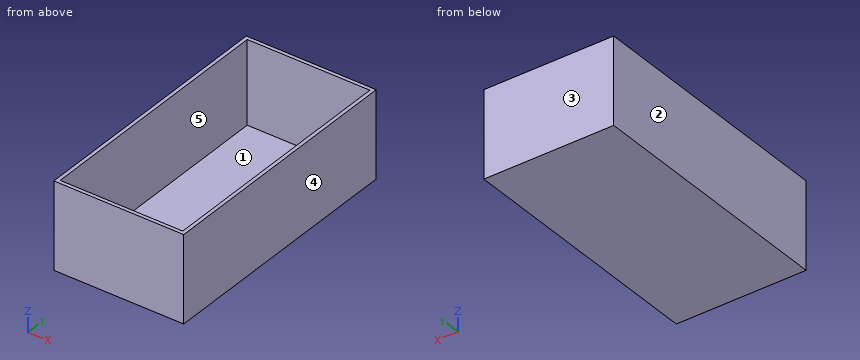
Autodesk Inventor part; units mm, degrees
ref_plane "YZ Plane" through (0, 0, 0) normal (1, 0, 0) x (0, 1, 0)
ref_plane "XZ Plane" through (0, 0, 0) normal (0, 1, 0) x (-1, 0, 0)
ref_plane "XY Plane" through (0, 0, 0) normal (0, 0, 1) x (1, 0, 0)
sketch "grey cabinet" plane through (0, 0, 0) normal (0, 1, 0) x (-1, 0, 0)
  line L0 (914.4, 609.6) -> (0, 609.6)
  line L1 (0, 609.6) -> (0, 0)
  line L2 (0, 0) -> (914.4, 0)
  line L3 (914.4, 0) -> (914.4, 609.6)
  dimension "d0" = 914.4
  dimension "d1" = 609.6
extrude "grey cabinet2" add sketch "grey cabinet" along normal blind 1828.8
shell "Shell1" thickness 25.4 removed faces 1 at (-609.6, 609.6, 609.6)
properties part number "grey cabinet"
Can you work these out from the model? Positions are in its coordinate system, mm. Face numbers are marked on the shaded views. A direction names the side the tool comes from. Round coordinates to 2 decimals unless told otherwise and drop trailing zeros. Loops run counter-clockwise (first coordinate to the right, second up) from the corner with the lowest first, then second, coordinate; pieces in that order, holes last. Notation, with made-up numbers: (-7, 49.25) -> (46, 49.25) arc R20 ccw to (46, 60.25) -> close; hole circle Ø7 at (-39, 52). An arc over 180 degrees is marked (long way). One line per item, written item: value. Start each with the question number.
1. If we section it at C-C, the plane x = -718: Write out the boundary of the cut face in (y, z), then the cut area to 3 significant figures.
2. If we section it at A-A, the plane z = 543.5: Write out the boundary of the cut face in (x, y).
3. If I drill on probe 1 along X at (y, z) = (388.5, 225.5); probe 2 along Y at (x, z) = (-160.5, 513); probe 3 along Z at (x, y) = (-839.5, 1678), over which ranges is the centre line in solid material (lowest first)?
4. If we section it at B-B, the plane y = 1454: Write out the boundary of the cut face in (x, z), then the cut area to 3 significant figures.
5. If we mould it in two halves opening along Y, with no side actions, what happens to the marked faces 1, 2 and 3? For each: pulls with the +Y half, pulls with the -Y half, needs draft (parallel to the pull), parting line crosses it, or undercut.
6. For pin 1 (5 mm diameter, centred on x = -574, z = 324, fed in from -Y), with a flat end and sliding along its axis, tell me the tip position at first contact or that it passes through.
7. For the marked faces 4 and 5, which set-ups out of +Z, -Z, +X, -X, +Y, -Y let a thin tool reach every point of the face, with its end or its side?
Calculated:
1. outline: (0, 0) -> (1828.8, 0) -> (1828.8, 609.6) -> (1803.4, 609.6) -> (1803.4, 25.4) -> (25.4, 25.4) -> (25.4, 609.6) -> (0, 609.6) -> close
1. area: 76,100 mm²
2. outline: (-914.4, 0) -> (0, 0) -> (0, 1828.8) -> (-914.4, 1828.8) -> close; hole (-889, 25.4) -> (-25.4, 25.4) -> (-25.4, 1803.4) -> (-889, 1803.4) -> close
3. probe 1: x = -914.4 to -889, -25.4 to 0
3. probe 2: y = 0 to 25.4, 1803.4 to 1828.8
3. probe 3: z = 0 to 25.4
4. outline: (-914.4, 0) -> (0, 0) -> (0, 609.6) -> (-25.4, 609.6) -> (-25.4, 25.4) -> (-889, 25.4) -> (-889, 609.6) -> (-914.4, 609.6) -> close
4. area: 52,900 mm²
5. face 1: undercut
5. face 2: needs draft
5. face 3: pulls with the +Y half
6. pin 1: stops at y = 0
7. face 4: +Z, -Z, +X, +Y, -Y
7. face 5: +Z
